Geometry check sheet. Reference: the model listing, model coordinates, mm. A direction names the side the tool comes from. Coordinates: 2 decimals unless noted, no trailing zeros. Order: outer loops, then holes, each group sorted by start corner. A loop starts at its lowest first (then second) coordinate and runs counter-clockwise, first axis right, second up.
```python
from build123d import *

# Parameters (mm, degrees)
SKETCH1_R           = 40
BOSS_EXTRUDE1_DEPTH = 5
SKETCH1_5_R         = 3
CUT_EXTRUDE3_DEPTH  = 5
SKETCH1_8_R         = 15.5
BOSS_EXTRUDE2_DEPTH = 6
CHAMFER1_SIZE       = 1
SKETCH1_20_R        = 1.4
CUT_EXTRUDE12_DEPTH = 7
SKETCH1_22_R        = 2.75
CUT_EXTRUDE13_DEPTH = 3


with BuildPart() as part:
    # Sketch1 → Boss-Extrude1 (new body)
    with BuildSketch(Plane.XY):
        Circle(SKETCH1_R)
    extrude(amount=BOSS_EXTRUDE1_DEPTH)

    # Sketch1<5> → Cut-Extrude3 (cut)
    with BuildSketch(Plane.XY):
        with Locations((-17.67766953, 17.67766953)):
            Circle(SKETCH1_5_R)
        with Locations((17.67766953, 17.67766953)):
            Circle(SKETCH1_5_R)
        with Locations((17.67766953, -17.67766953)):
            Circle(SKETCH1_5_R)
        with Locations((-17.67766953, -17.67766953)):
            Circle(SKETCH1_5_R)
    extrude(amount=CUT_EXTRUDE3_DEPTH, mode=Mode.SUBTRACT)

    # Sketch1<8> → Boss-Extrude2 (add)
    with BuildSketch(Plane.XY):
        Circle(SKETCH1_8_R)
    extrude(amount=-BOSS_EXTRUDE2_DEPTH)

    # Chamfer1
    chamfer1_edges = [part.edges().sort_by_distance(p)[0] for p in [
        (-15.5, 0, -6),
    ]]
    chamfer(chamfer1_edges, length=CHAMFER1_SIZE)

    # Sketch1<20> → Cut-Extrude12 (cut)
    with BuildSketch(Plane.XY):
        with Locations((-20.57248383, 28.315594803)):
            Circle(SKETCH1_20_R)
        with Locations((20.57248383, 28.315594803)):
            Circle(SKETCH1_20_R)
        with Locations((33.28697807, 10.815594803)):
            Circle(SKETCH1_20_R)
        with Locations((33.28697807, -10.815594803)):
            Circle(SKETCH1_20_R)
        with Locations((20.57248383, -28.315594803)):
            Circle(SKETCH1_20_R)
        with Locations((-20.57248383, -28.315594803)):
            Circle(SKETCH1_20_R)
        with Locations((-33.28697807, -10.815594803)):
            Circle(SKETCH1_20_R)
        with Locations((-33.28697807, 10.815594803)):
            Circle(SKETCH1_20_R)
    extrude(amount=CUT_EXTRUDE12_DEPTH, mode=Mode.SUBTRACT)

    # Sketch1<22> → Cut-Extrude13 (cut)
    with BuildSketch(Plane.XY):
        with Locations((20.57248383, 28.315594803)):
            Circle(SKETCH1_22_R)
        with Locations((33.28697807, 10.815594803)):
            Circle(SKETCH1_22_R)
        with Locations((33.28697807, -10.815594803)):
            Circle(SKETCH1_22_R)
        with Locations((20.57248383, -28.315594803)):
            Circle(SKETCH1_22_R)
        with Locations((-20.57248383, -28.315594803)):
            Circle(SKETCH1_22_R)
        with Locations((-33.28697807, -10.815594803)):
            Circle(SKETCH1_22_R)
        with Locations((-33.28697807, 10.815594803)):
            Circle(SKETCH1_22_R)
        with Locations((-20.57248383, 28.315594803)):
            Circle(SKETCH1_22_R)
    extrude(amount=CUT_EXTRUDE13_DEPTH, mode=Mode.SUBTRACT)


solid = part.part
```
Item 1: Release check for a two-part mould opening along X. For faces 3 (the face through (-8.67, -39.05, 2.46)), 4 (the face through (-1, -17, 0)), 5 (the face through (35.827, 9.762, 1.479)) record: pulls with the +X half, pulls with the -X half, needs draft (parallel to the pull), parting line crosses it, or undercut.
Item 2: Sectioned sample at C-C (z = -3.5). Record the cut outline in (x, y), and give its area (3 significant figures).
Item 3: Sectioned sample at A-A (y = 0). Record the cut outline in (x, z).
Item 4: Depth check by flat-ended pin: P1, Ø2, axis at x = 33.29, y = 10.82, coming from the +Z side; P2, Ø5, axis at x = 25.5, z = 2, coming from the -Y side; P3, Ø4.5, axis at x = -20.57, y = -28.32, coming from the -Z side; P4, Ø6, axis at x = 32, y = -10, coming from the -Z side. Enter the tip coordinate at first touch or a pass-through.
Item 5: Sectioned sample at D-D (y = 24.5). Record the cut outline in (x, z).
Item 6: Thickness scan on line 1 along Z through (x, y) = (36, 0.5); line 2 along Y through (x, z) = (5, -3.25); line 3 along Y through (x, z) = (35.5, 0.75). Record the ranges inside material, lowest first.
Item 7: Tool access check on faces 1 (the face through (-35, 11, 3)), 2 (the face through (21.218, 27.074, 3.986)). Record the directions out of +Z, -Z, +X, -X, +Y, -Y that give a thin tool (end or side, any length) a straight path to the whole face; none if there is none.
Geometry check:
1. face 3: parting line crosses it
1. face 4: needs draft
1. face 5: undercut
2. outline: circle Ø31 at (0, 0)
2. area: 755 mm2
3. outline: (-40, 0) - (-15.5, 0) - (-15.5, -5) - (-14.5, -6) - (14.5, -6) - (15.5, -5) - (15.5, 0) - (40, 0) - (40, 5) - (-40, 5) - close
4. P1: passes through
4. P2: stops at y = -32.73
4. P3: stops at z = 3
4. P4: stops at z = 0
5. outline: (-31.62, 0) - (31.62, 0) - (31.62, 5) - (-31.62, 5) - close
6. line 1: z = 0 to 5
6. line 2: y = -14.67 to 14.67
6. line 3: y = -18.43 to -12.45, -9.18 to 9.18, 12.45 to 18.43
7. face 1: -Z
7. face 2: +Z, -Z
